from build123d import *

# Parameters (mm, degrees)
SKETCH1_W                   = 38.1
SKETCH1_H                   = 76.2
BOSS_EXTRUDE1_DEPTH         = 31.75
SKETCH3_W                   = 25.4
SKETCH3_H                   = 76.2
CUT_EXTRUDE2_DEPTH          = 31.75
SKETCH4_W                   = 25.4
SKETCH4_H                   = 25.4
CUT_EXTRUDE3_DEPTH          = 89.44526556
SKETCH5_W                   = 31.75
SKETCH5_H                   = 6.35
BOSS_EXTRUDE2_DEPTH         = 50.8
SKETCH6_R                   = 3.175
CUT_EXTRUDE4_DEPTH          = 50.8
FILLET2_R                   = 9.525
SKETCH7_W                   = 31.75
SKETCH7_H                   = 19.05
BOSS_EXTRUDE3_DEPTH         = 6.35
SKETCH11_W                  = 38.1
SKETCH11_H                  = 6.35
BOSS_EXTRUDE4_DEPTH         = 12.7
F_1_4_20_TAPPED_HOLE2_D     = 5.1054
F_1_4_20_TAPPED_HOLE2_DEPTH = 16.51
F_1_4_20_TAPPED_HOLE2_TIP   = 1.533816902


with BuildPart() as part:
    # Sketch1 → Boss-Extrude1 (new body)
    with BuildSketch(Plane.XY):
        with Locations((19.05, 38.1)):
            Rectangle(SKETCH1_W, SKETCH1_H)
    extrude(amount=-BOSS_EXTRUDE1_DEPTH)

    # Sketch3 → Cut-Extrude2 (cut)
    with BuildSketch(Plane.ZY):
        with Locations((-19.05, 38.1)):
            Rectangle(SKETCH3_W, SKETCH3_H)
    extrude(amount=-CUT_EXTRUDE2_DEPTH, mode=Mode.SUBTRACT)

    # Sketch4 → Cut-Extrude3 (cut, through all)
    with BuildSketch(Plane.ZY.offset(-31.75)):
        with Locations((-19.05, 12.7)):
            Rectangle(SKETCH4_W, SKETCH4_H)
    extrude(amount=-CUT_EXTRUDE3_DEPTH, mode=Mode.SUBTRACT)

    # Sketch5 → Boss-Extrude2 (add)
    with BuildSketch(Plane(origin=(0, 76.2, 0), x_dir=(1, 0, 0), z_dir=(0, 1, 0))):
        with Locations((15.875, 28.575)):
            Rectangle(SKETCH5_W, SKETCH5_H)
    extrude(amount=-BOSS_EXTRUDE2_DEPTH)

    # Sketch6 → Cut-Extrude4 (cut)
    with BuildSketch(Plane(origin=(0, 0, -31.75), x_dir=(-1, 0, 0), z_dir=(0, 0, -1))):
        with Locations((-6.35, 63.5)):
            Circle(SKETCH6_R)
    extrude(amount=-CUT_EXTRUDE4_DEPTH, mode=Mode.SUBTRACT)

    # Fillet2
    fillet2_edges = [part.edges().sort_by_distance(p)[0] for p in [
        (0, 76.2, -3.175),
        (0, 76.2, -28.575),
    ]]
    fillet(fillet2_edges, radius=FILLET2_R)

    # Sketch7 → Boss-Extrude3 (add)
    with BuildSketch(Plane(origin=(0, 25.4, 0), x_dir=(-1, 0, 0), z_dir=(0, -1, 0))):
        with Locations((-15.875, 15.875)):
            Rectangle(SKETCH7_W, SKETCH7_H)
    extrude(amount=-BOSS_EXTRUDE3_DEPTH)

    # Sketch11 → Boss-Extrude4 (add)
    with BuildSketch(Plane.XZ):
        with Locations((19.05, -3.175)):
            Rectangle(SKETCH11_W, SKETCH11_H)
    extrude(amount=BOSS_EXTRUDE4_DEPTH)

    # 1/4-20 Tapped Hole2
    with Locations(Plane(origin=(9.525, -3.175, 0), x_dir=(1, 0, 0), z_dir=(0, 0, 1))):
        with Locations((0, 0), (19.05, 0), (0, 19.05), (19.05, 19.05)):
            Hole(F_1_4_20_TAPPED_HOLE2_D / 2, depth=F_1_4_20_TAPPED_HOLE2_DEPTH)
            with Locations((0, 0, -(F_1_4_20_TAPPED_HOLE2_DEPTH + F_1_4_20_TAPPED_HOLE2_TIP / 2))):  # 118° drill point
                Cone(0, F_1_4_20_TAPPED_HOLE2_D / 2, F_1_4_20_TAPPED_HOLE2_TIP, mode=Mode.SUBTRACT)


solid = part.part
Here's how the part is built. I have some questions about the finished solid (model axes, mm). A direction names the side the tool comes from. Give positions to 0.01 mm unless a question says otherwise; leave off trailing zeros. Order: outer loops, then holes, each group sorted by start corner. A loop starts at its lowest first (then second) coordinate and runs counter-clockwise, first axis right, second up. Notation, with made-up numbers: M 18,73.5 L 43,73.5 A17 cw 43,96.5 Z; hole C 88.25,-4 d8. An arc over 180 degrees is marked long. Answer as a JSON object with one key per item and string values. Group by question number.
1) Please list where these lines run through material, in increasing order: L1, parallel to Z at x = 2, y = 61.5; L2, parallel to Y at x = 33.5, z = -26.5; L3, parallel to Z at x = 26, y = 0.5. Write a range as [from, to].
2) Suppose I cut it at A-A, the plane y = 63.5. Write out the boundary of the cut face in (x, z) (3 decimals).
3) I'm going to push flat-ended pins straight in: pin 1 Ø15 at (y, z) = (59.5, -13.5) entering from -X; pin 2 Ø5 at (x, z) = (5, -19) entering from +Y; pin 3 Ø19 at (x, y) = (21, 5) entering from -Z; pin 4 Ø8 at (x, z) = (17.5, -18.5) entering from -Y. Where does each tip first touch, or does it pass through?
4) Suppose I cut it at C-C, the plane x = 15. Write out the boundary of the cut face in (y, z).
5) We'd pull the mould along Z, two halves only. Please class faces 4 (the flat face through (16, 31.75, -16)), 5 (the cylindrical face through (4.643, 66.177, -28.619)), 6 (the flat face through (19, 7, -6.35)), 7 (the flat face through (19, 32, 0)): pulls with the +Z half, pulls with the -Z half, needs draft (parallel to the pull), parting line crosses it, or undercut.
6) Suppose I cut it at B-B, the plane z = -28. Write out the boundary of the cut face in (x, y) (3 decimals), plus the area to 3 significant figures.
7) Suppose I cut it at D-D, the plane y = 47.5. Write out the boundary of the cut face in (x, z), plus the area to 3 significant figures.
8) On a 3-axis mill with a long thin cutter (end or side, diameter ignored), from which of +Z, -Z, +X, -X, +Y, -Y can I reach the whole of each face in a straight line? I mean faces 1 (the flat face through (31.75, 54, -16)), 2 (the flat face through (38.1, 42, -13)), 3 (the flat face through (19, 25.4, -19)). Say none if no direction works.
Results found:
{
 "1": {"L1": "[-31.75, -25.4], [-6.35, 0]", "L2": "[25.4, 76.2]", "L3": "[-6.35, 0]"},
 "2": {"outline": "M 0,-31.75 L 3.175,-31.75 L 3.175,-25.4 L 0,-25.4 Z; M 0,-6.35 L 3.175,-6.35 L 3.175,0 L 0,0 Z; M 9.525,-31.75 L 38.1,-31.75 L 38.1,0 L 9.525,0 L 9.525,-6.35 L 31.75,-6.35 L 31.75,-25.4 L 9.525,-25.4 Z"},
 "3": {"pin 1": "x = 0", "pin 2": "y = 31.75", "pin 3": "z = -6.35", "pin 4": "y = 25.4"},
 "4": {"outline": "M -12.7,-6.35 L 25.4,-6.35 L 25.4,-31.75 L 76.2,-31.75 L 76.2,-25.4 L 31.75,-25.4 L 31.75,-6.35 L 76.2,-6.35 L 76.2,0 L -12.7,0 Z"},
 "5": {"face 4": "undercut", "face 5": "needs draft", "face 6": "pulls with the -Z half", "face 7": "pulls with the +Z half"},
 "6": {"outline": "M 0,25.4 L 38.1,25.4 L 38.1,76.2 L 9.525,76.2 A9.525 ccw 0,66.675 Z; hole C 6.35,63.5 d6.35", "area": "1,880 mm²"},
 "7": {"outline": "M 0,-31.75 L 38.1,-31.75 L 38.1,0 L 0,0 L 0,-6.35 L 31.75,-6.35 L 31.75,-25.4 L 0,-25.4 Z", "area": "605 mm²"},
 "8": {"face 1": "-X, +Y", "face 2": "+Z, -Z, +X, +Y, -Y", "face 3": "-Z, +X, -X, -Y"}
}
